```python
from build123d import *

# Parameters (mm, degrees)
ESBO_O2_R                = 2.95
RESSALTO_EXTRUS_O1_DEPTH = 8
ESBO_O3_R                = 4.076601305
ESBO_O3_R_2              = 1.475
RESSALTO_EXTRUS_O2_DEPTH = 1.2


with BuildPart() as part:
    # Esboço2 → Ressalto-extrusão1 (new body)
    with BuildSketch(Plane.XY):
        Circle(ESBO_O2_R)
        with BuildLine():
            Line((1.95, -2.00935313), (1.95, 2.00935313))
            ThreePointArc((1.95, 2.00935313), (0, 2.8), (-1.95, 2.00935313))
            Line((-1.95, 2.00935313), (-1.95, -2.00935313))
            ThreePointArc((-1.95, -2.00935313), (0, -2.8), (1.95, -2.00935313))
        make_face(mode=Mode.SUBTRACT)
    extrude(amount=RESSALTO_EXTRUS_O1_DEPTH)

    # Esboço3 → Ressalto-extrusão2 (add)
    with BuildSketch(Plane(origin=(0, 0, 0), x_dir=(-1, 0, 0), z_dir=(0, 0, -1))):
        Circle(ESBO_O3_R)
        Circle(ESBO_O3_R_2, mode=Mode.SUBTRACT)
    extrude(amount=RESSALTO_EXTRUS_O2_DEPTH)


solid = part.part
```
For this review, take the finished solid that the model builds, in its own axes (mm). A direction names the side the tool comes from. Round coordinates to 2 decimals unless told otherwise and drop trailing zeros. Loops run counter-clockwise (first coordinate to the right, second up) from the corner with the lowest first, then second, coordinate; pieces in that order, holes last.
Q1. Mouldability with a two-part tool opening along X and no side actions: class faces 1 (the face through (1.76, 0.04, 0)), 2 (the face through (0, -2, -1.2)), 3 (the face through (-2.947, 0.13, 3.944)) as +X half, -X half, draft (parallel to the pull), parting line (faces both ways), or undercut.
Result sheet:
face 1: undercut
face 2: draft
face 3: parting line
Q2. Add section D-D on y = -2.5. Write out the cut boundary in (x, z), plus the area to 3 significant figures.
Result sheet:
outline: (-3.22, -1.2) - (3.22, -1.2) - (3.22, 0) - (1.57, 0) - (1.57, 8) - (1.26, 8) - (1.26, 0) - (-1.26, 0) - (-1.26, 8) - (-1.57, 8) - (-1.57, 0) - (-3.22, 0) - close
area: 12.6 mm2
Q3. Add section B-B on x = 0. Write out the cut boundary in (y, z) (3 decimals), plus the area to 3 significant figures.
Result sheet:
outline: (-4.077, -1.2) - (-1.475, -1.2) - (-1.475, 0) - (-2.8, 0) - (-2.8, 8) - (-2.95, 8) - (-2.95, 0) - (-4.077, 0) - close; (1.475, -1.2) - (4.077, -1.2) - (4.077, 0) - (2.95, 0) - (2.95, 8) - (2.8, 8) - (2.8, 0) - (1.475, 0) - close
area: 8.64 mm2
Q4. Add section C-C on z = 3.5. Write out the cut boundary in (x, y), plus the area to 3 significant figures.
Result sheet:
outline: circle Ø5.9 at (0, 0); hole (-1.95, -2.01) arc R2.8 ccw to (1.95, -2.01) - (1.95, 2.01) arc R2.8 ccw to (-1.95, 2.01) - close
area: 7.42 mm2
Q5. To check wall thickness, follow line 1 along Y through (x, z) = (0, -0.35) (3 decimals); line 2 along X through (y, z) = (1.25, 1.75); line 3 along X through (y, z) = (-1.75, 1.25). State the ranges of each line that lie inside material, in increasing order.
Result sheet:
line 1: y = -4.077 to -1.475, 1.475 to 4.077
line 2: x = -2.67 to -1.95, 1.95 to 2.67
line 3: x = -2.37 to -1.95, 1.95 to 2.37
Q6. Machinability: for faces 4 (the face through (1.95, 0, 4)), 5 (the face through (1.474, 0.065, -0.592)), which of the approach directions +Z, -Z, +X, -X, +Y, -Y give a long, thin tool a straight path to every point of the face, cutting with its end or side? Answer none if there is none.
Result sheet:
face 4: +Z
face 5: +Z, -Z
Q7. Insertion check: pin 1 Ø1.5 at (x, z) = (2, 2.5) entering from +Y; pin 2 Ø4.5 at (y, z) = (0, 2.5) entering from +X; pin 3 Ø2 at (x, y) = (0.5, -0.5) entering from +Z. Each pin has a flat end and moves straight along its axis. Give the tip position at first contact, or say it passes through.
Result sheet:
pin 1: stops at y = 2.67
pin 2: stops at x = 2.95
pin 3: stops at z = 0
Q8. Add section A-A on y = 0. Write out the cut boundary in (x, z) (3 decimals).
Result sheet:
outline: (-4.077, -1.2) - (-1.475, -1.2) - (-1.475, 0) - (-1.95, 0) - (-1.95, 8) - (-2.95, 8) - (-2.95, 0) - (-4.077, 0) - close; (1.475, -1.2) - (4.077, -1.2) - (4.077, 0) - (2.95, 0) - (2.95, 8) - (1.95, 8) - (1.95, 0) - (1.475, 0) - close
